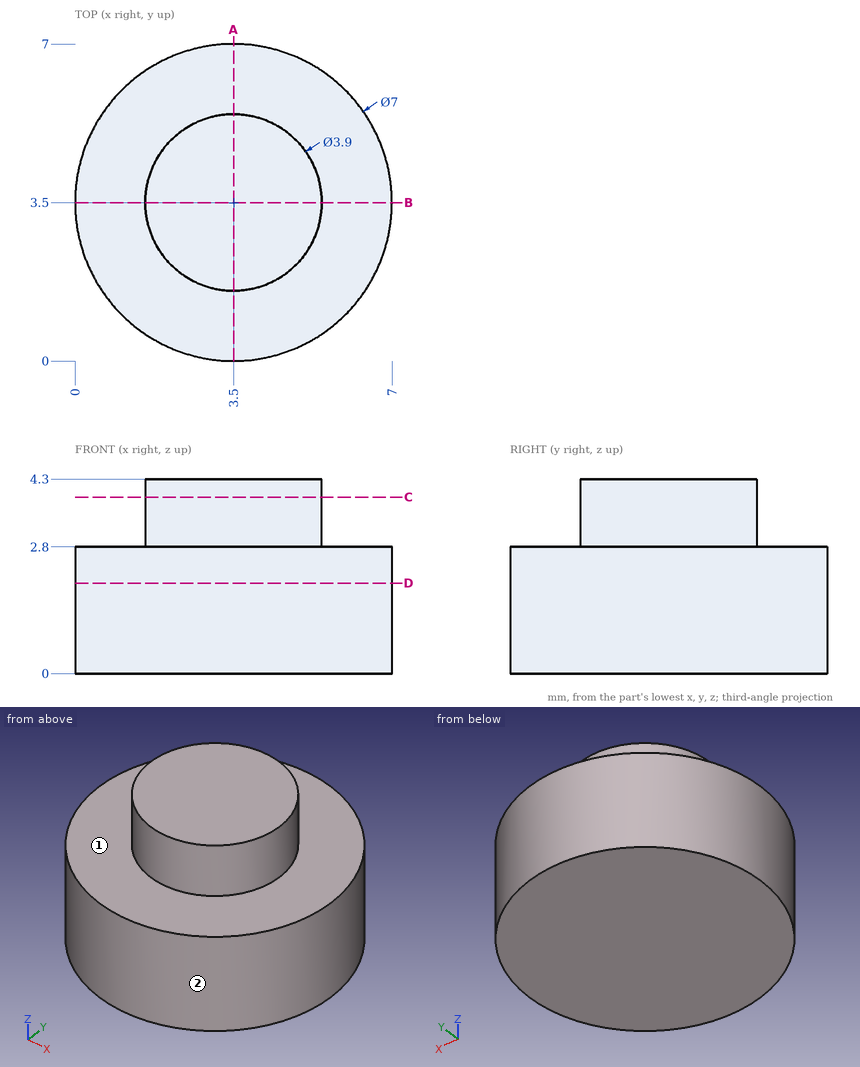
Answer from the drawing. Dimensions are ordinates in mm from the lowest x, y and z of the part. A direction names the side the tool comes from. Give positions to 0.01 mm unless a question says otherwise; leave off trailing zeros. Loops run counter-clockwise (first coordinate to the right, second up) from the corner with the lowest first, then second, coordinate; pieces in that order, holes last.
Item 1: The part is cut by section A-A (x = 3.5). Write down the section's boundary in (y, z).
Item 2: This flat-tipped pin is pushed along its axis until it touches: pin 1 Ø1.5 at (y, z) = (5, 1.5) entering from -X. Where does it stop, or does it pass through?
Item 3: For the marked faces 1 and 2, determine the directions among +Z, -Z, +X, -X, +Y, -Y from which every point of the face is accessible in a straight line to the end or side of a thin tool.
Item 4: The part is cut by section C-C (z = 3.9). Write down the section's boundary in (x, y).
Item 5: Find the intervals of material crossed by line 1 along Z through (x, y) = (2, 2); line 2 along Y through (x, z) = (3.5, 3.9); line 3 along Y through (x, z) = (2.5, 1.25), in increasing order.
Item 6: The part is cut by section D-D (z = 2). Write down the section's boundary in (x, y), and give its area (3 significant figures).
Taken from the geometry:
1. outline: (0, 0) - (7, 0) - (7, 2.8) - (5.45, 2.8) - (5.45, 4.3) - (1.55, 4.3) - (1.55, 2.8) - (0, 2.8) - close
2. pin 1: stops at x = 0.08
3. face 1: +Z
3. face 2: +Z, -Z
4. outline: circle Ø3.9 at (3.5, 3.5)
5. line 1: z = 0 to 2.8
5. line 2: y = 1.55 to 5.45
5. line 3: y = 0.15 to 6.85
6. outline: circle Ø7 at (3.5, 3.5)
6. area: 38.5 mm2
